For this review, take the finished solid that the model builds, in its own axes (mm). Face numbers are marked on the shaded views. Coordinates: 2 decimals unless noted, no trailing zeros. Loops run counter-clockwise (first coordinate to the right, second up) from the corner with the lowest first, then second, coordinate; pieces in that order, holes last. Notation, with made-up numbers: (61, 16) -> (113, 16) arc R28 cw to (113, 39) -> close; hole circle Ø9 at (78, -24.75). An arc over 180 degrees is marked (long way). Use a Markdown table: item, result.
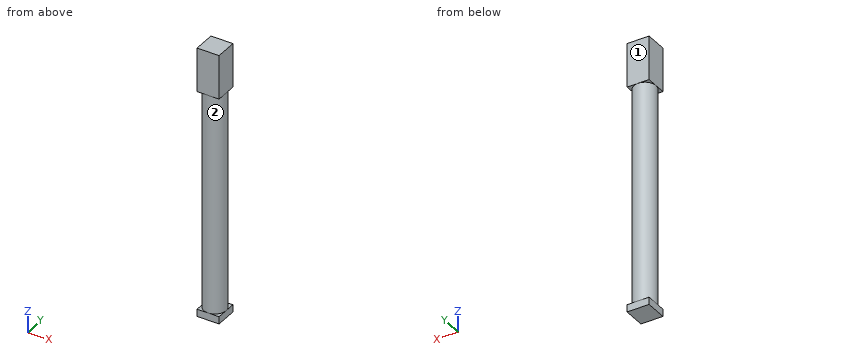
from build123d import *

# Parameters (mm, degrees)
SKETCH1_R           = 1.905
BOSS_EXTRUDE1_DEPTH = 19.05
SKETCH2_W           = 3.81
SKETCH2_H           = 3.81
BOSS_EXTRUDE2_DEPTH = 7.62
SKETCH3_W           = 3.81
SKETCH3_H           = 3.81
BOSS_EXTRUDE3_DEPTH = 1.27


with BuildPart() as part:
    # Sketch1 → Boss-Extrude1 (new, symmetric)
    with BuildSketch(Plane.XY):
        with Locations(Location((0, 0, 0), (0, 0, 180))):
            Circle(SKETCH1_R)
    extrude(amount=BOSS_EXTRUDE1_DEPTH, both=True)

    # Sketch2 → Boss-Extrude2 (add)
    with BuildSketch(Plane.XY.offset(19.05)):
        Rectangle(SKETCH2_W, SKETCH2_H)
    extrude(amount=BOSS_EXTRUDE2_DEPTH)

    # Sketch3 → Boss-Extrude3 (add)
    with BuildSketch(Plane(origin=(0, 0, -19.05), x_dir=(-1, 0, 0), z_dir=(0, 0, -1))):
        Rectangle(SKETCH3_W, SKETCH3_H)
    extrude(amount=BOSS_EXTRUDE3_DEPTH)


solid = part.part
(1) For line 1 along Z through (x, y) = (-1.4, -1.45); line 2 along Y through (x, z) = (-1.4, 10.5); line 3 along Y through (x, z) = (0.15, 1), list the stretches that pass through material, from the lowest coordinate up.
Found:
| item | result |
|---|---|
| line 1 | z = -20.32 to -19.05, 19.05 to 26.67 |
| line 2 | y = -1.29 to 1.29 |
| line 3 | y = -1.9 to 1.9 |
(2) Mouldability with a two-part tool opening along Z and no side actions: class the marked faces 1 and 2 as pulls with the +Z half, pulls with the -Z half, needs draft (parallel to the pull), parting line crosses it, or undercut.
Found:
| item | result |
|---|---|
| face 1 | needs draft |
| face 2 | undercut |
(3) Take a section at A-A on x = -1.2. Write out the cut boundary in (y, z) (3 decimals).
Found:
| item | result |
|---|---|
| outline | (-1.905, -20.32) -> (1.905, -20.32) -> (1.905, -19.05) -> (1.48, -19.05) -> (1.48, 19.05) -> (1.905, 19.05) -> (1.905, 26.67) -> (-1.905, 26.67) -> (-1.905, 19.05) -> (-1.48, 19.05) -> (-1.48, -19.05) -> (-1.905, -19.05) -> close |
(4) Take a section at B-B on y = -0.9. Write out the cut boundary in (x, z) (3 decimals).
Found:
| item | result |
|---|---|
| outline | (-1.905, -20.32) -> (1.905, -20.32) -> (1.905, -19.05) -> (1.679, -19.05) -> (1.679, 19.05) -> (1.905, 19.05) -> (1.905, 26.67) -> (-1.905, 26.67) -> (-1.905, 19.05) -> (-1.679, 19.05) -> (-1.679, -19.05) -> (-1.905, -19.05) -> close |
(5) Take a section at C-C on z = 2. Write out the cut boundary in (x, y) (3 decimals).
Found:
| item | result |
|---|---|
| outline | circle Ø3.81 at (0, 0) |
(6) For pin 1 Ø2 at (y, z) = (-1.5, 3.5) entering from +X, flat-tipped, find the tip position at first contact; note if it passes through.
Found:
| item | result |
|---|---|
| pin 1 | stops at x = 1.84 |
